Here's the drawing with two shaded views (mm, measured from the low corner). I have some questions. A direction names the side the tool comes from. Give positions to 0.01 mm unless a question says otherwise; leave off trailing zeros. Write each loop counter-clockwise with the first axis right and the second up, starting at its lowest first coordinate (ties: lowest second). Pieces come first, ordered by that corner, then holes. Notation, with made-up numbers: M 5,-6 L 24,-6 A6 ccw 24,5 Z; hole C 74.5,55.25 d7. An arc over 180 degrees is marked long. Use one line per item in the form item = value. Start each with the question number.
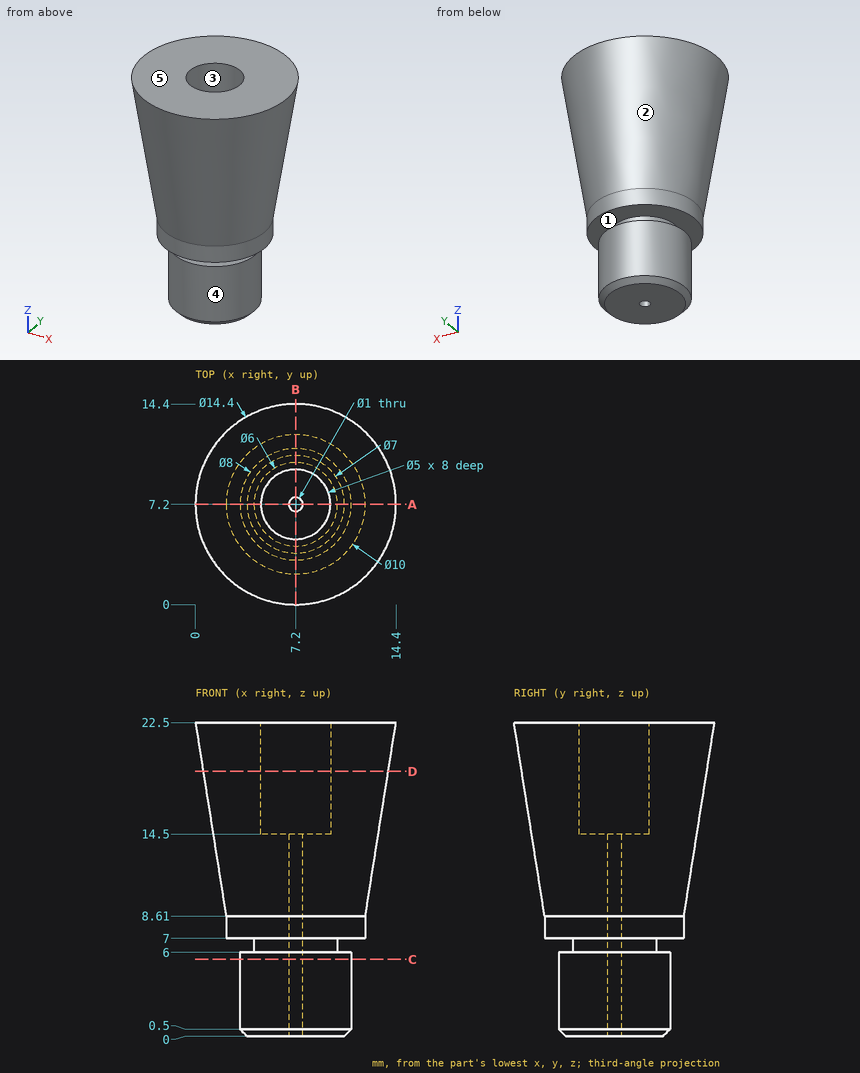
1) Suppose I cut it at A-A, the plane y = 7.2. List the corners of the cut face in (x, z) for me, and give its area (3 significant figures).
2) On a 3-axis mill with a long thin cutter (end or side, diameter ignored), from which of +Z, -Z, +X, -X, +Y, -Y can I reach the whole of each face in a straight line? I mean the marked faces 4 and 5. Say none if no direction works.
3) Thinking about a two-plate mould opening in Y: for the marked faces 1, 2 and 3, which applies, released by +Y, released by -Y, zero draft, split by the parting line, or undercut?
4) Suppose I cut it at C-C, the plane z = 5.5. List the corners of the cut face in (x, y) for me.
5) Please list where these lines run through material, in increasing order: line 1 (Y direction, x = 7.2, z = 3.75); line 2 (Y direction, x = 7.25, z = 7.5); line 3 (Z direction, x = 7.25, y = 5.75).
6) Will these pins go through, and if not, where does the flat tip stop? P1, Ø3, axis at x = 8, z = 17, coming from the -Y side; P2, Ø1.5, axis at x = 10.5, z = 13.5, coming from the +Y side; P3, Ø4, axis at x = 7, y = 5.5, coming from the +Z side; P4, Ø6, axis at y = 9, z = 7.5, coming from the +X side.
7) Suppose I cut it at D-D, the plane z = 19. List the corners of the cut face in (x, y) for me.
Checks:
q1.outline = M 0,22.5 L 2.2,8.61 L 2.2,7 L 4.2,7 L 4.2,6 L 3.2,6 L 3.2,0.5 L 3.7,0 L 6.7,0 L 6.7,14.5 L 4.7,14.5 L 4.7,22.5 Z; M 7.7,0 L 10.7,0 L 11.2,0.5 L 11.2,6 L 10.2,6 L 10.2,7 L 12.2,7 L 12.2,8.61 L 14.4,22.5 L 9.7,22.5 L 9.7,14.5 L 7.7,14.5 Z
q1.area = 185 mm^2
q2.face_4 = -Z
q2.face_5 = +Z, +X, -X, +Y, -Y
q3.face_1 = zero draft
q3.face_2 = split by the parting line
q3.face_3 = undercut
q4.outline = C 7.2,7.2 d8; hole C 7.2,7.2 d1
q5.line_1 = 3.2 to 6.7, 7.7 to 11.2
q5.line_2 = 2.2 to 6.7, 7.7 to 12.2
q5.line_3 = 0 to 14.5
q6.P1 = 0.65
q6.P2 = 12.4
q6.P3 = 22.5
q6.P4 = 12.43
q7.outline = C 7.2,7.2 d13.29; hole C 7.2,7.2 d5
